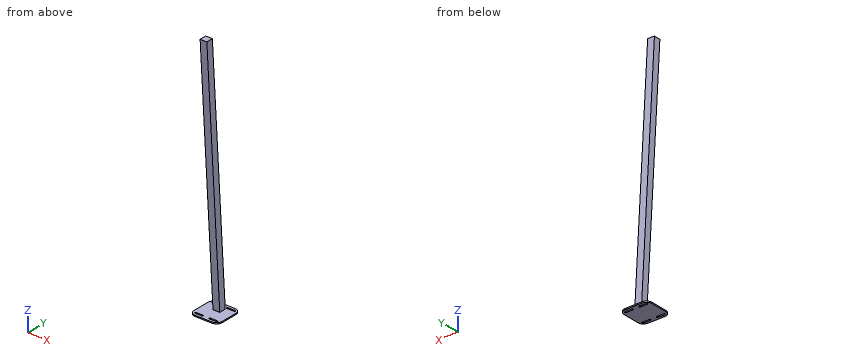
from build123d import *

# Parameters (mm, degrees)
F1_DEPTH = 10
F2_W     = 60
F2_H     = 60


with BuildPart() as f1:
    # F0 (on Top) → F1 (new body)
    with BuildSketch(Plane.XY):
        with BuildLine():
            Line((-200, 0), (-50, 0))
            ThreePointArc((-50, 0), (-14.6446609407, 14.6446609407), (0, 50))
            Line((0, 50), (0, 200))
            ThreePointArc((0, 200), (-14.6446609407, 235.3553390593), (-50, 250))
            Line((-50, 250), (-200, 250))
            ThreePointArc((-200, 250), (-235.3553390593, 235.3553390593), (-250, 200))
            Line((-250, 200), (-250, 50))
            ThreePointArc((-250, 50), (-235.3553390593, 14.6446609407), (-200, 0))
        make_face()
        with BuildLine():
            ThreePointArc((-221, 22), (-228, 29), (-221, 36))
            Line((-221, 36), (-157, 36))
            ThreePointArc((-157, 36), (-150, 29), (-157, 22))
            Line((-157, 22), (-221, 22))
        make_face(mode=Mode.SUBTRACT)
        with BuildLine():
            Line((-93, 36), (-29, 36))
            ThreePointArc((-29, 36), (-22, 29), (-29, 22))
            Line((-29, 22), (-93, 22))
            ThreePointArc((-93, 22), (-100, 29), (-93, 36))
        make_face(mode=Mode.SUBTRACT)
        with BuildLine():
            Line((-157, 214), (-221, 214))
            ThreePointArc((-221, 214), (-228, 221), (-221, 228))
            Line((-221, 228), (-157, 228))
            ThreePointArc((-157, 228), (-150, 221), (-157, 214))
        make_face(mode=Mode.SUBTRACT)
        with BuildLine():
            ThreePointArc((-93, 214), (-100, 221), (-93, 228))
            Line((-93, 228), (-29, 228))
            ThreePointArc((-29, 228), (-22, 221), (-29, 214))
            Line((-29, 214), (-93, 214))
        make_face(mode=Mode.SUBTRACT)
    extrude(amount=F1_DEPTH)

    # F4: sweep along a path in F3
    with BuildLine(Plane.YZ) as f4_path:
        Line((29, 2200), (170, 10))
    # F2 (on face) → F4 (sweep)
    with BuildSketch(Plane.XY.offset(10)):
        with Locations((-125, 170)):
            Rectangle(F2_W, F2_H)
    sweep(path=f4_path.line)


solid = f1.part
Source: CAD feature listing. Evaluate the final solid. Frame: model axes, mm. Give positions to 0.01 mm unless a question says otherwise; leave off trailing zeros. Write each loop counter-clockwise with the first axis right and the second up, starting at its lowest first coordinate (ties: lowest second). Pieces come first, ordered by that corner, then holes. Notation, with made-up numbers: (53.5, 22) -> (86.5, 22) arc R21 cw to (86.5, 36) -> close; hole circle Ø4 at (43.25, 31.25). An arc over 180 degrees is marked (long way). Return JSON: item names as keys, results as strings. Group by question number.
1. Section A-A, the plane z = 1087.5. Output: boundary loops of the cut face in (x, y), then the cut area to 3 significant figures.
2. Pin query (flat end, axial travel): pin 1 Ø3 at (x, z) = (-132, 1302.5) entering from -Y; pin 2 Ø8 at (x, z) = (-68, 7) entering from -Y; pin 3 Ø4 at (x, y) = (-176.5, 159.5) entering from -Z; pin 4 Ø2 at (x, y) = (-130, 215) entering from +Z. Return the tip coordinate at first contact, or that it passes through.
3. Material intervals for line 1 (Z direction, x = -231.5, y = 225); line 2 (X direction, y = 44.5, z = 1688.5); line 3 (Y direction, x = -124, z = 2000), sorted ascending. Write a range as from..to.
Determined:
{
 "1": {"outline": "(-155, 70.63) -> (-95, 70.63) -> (-95, 130.63) -> (-155, 130.63) -> close", "area": "3,600 mm2"},
 "2": {"pin 1": "stops at y = 56.69", "pin 2": "stops at y = 0", "pin 3": "stops at z = 0", "pin 4": "stops at z = 10"},
 "3": {"line 1": "z = 0..10", "line 2": "x = -155..-95", "line 3": "y = 11.88..71.88"}
}
